Input: part model. Units: mm. Frame: model coordinates. Face numbers are marked on the shaded views. A direction names the side the tool comes from. Coordinates: 2 decimals unless noted, no trailing zeros. Write each loop counter-clockwise with the first axis right and the second up, starting at its lowest first coordinate (ties: lowest second). Pieces come first, ordered by that corner, then holes.
1) Section query B-B (y = -48). Output: boundary loops of the cut face in (x, z).
2) Section query D-D (z = -57.5). Output: boundary loops of the cut face in (x, y), then the cut area to 3 significant figures.
3) Set-up query: the marked faces 4, 5, 6 and 7. Return all of +Z, -Z, +X, -X, +Y, -Y with unobstructed straight access to the full face (end or side cutting, diameter ignored); none if empty.
4) Pin query (flat end, axial travel): pin 1 Ø1.5 at (y, z) = (-69, 32) entering from -X; pin 2 Ø3.5 at (x, y) = (-122, -49.5) entering from -Z; pin 3 Ø10 at (x, y) = (22.5, -47) entering from -Z. Return the tip coordinate at first contact, or that it passes through.
5) Draft query along X for the marked faces 1, 2 and 3. Return one class per face: pulls with the +X half, pulls with the -X half, needs draft (parallel to the pull), parting line crosses it, or undercut.
6) Section query A-A (z = 0). State how many separate pieces and enclosed holes the cut face has, then the cut area to 3 significant figures.
7) Line query: L1, parallel to Z at x = 14, y = -43.5; L2, parallel to Y at x = -47.5, z = 53; L3, parallel to X at y = -43.5, z = -13.5. Output: solid intervals per line, ascending.
8) Section query C-C (x = 51.5). Output: boundary loops of the cut face in (y, z), then the cut area to 3 significant figures.
from build123d import *

# Parameters (mm, degrees)
SKETCH_6_W                     = 111
SKETCH_6_H                     = 9
SKETCH_7_W                     = 12
SKETCH_7_H                     = 30
EXTRUDE_5_DEPTH                = 30
SKETCH_8_R                     = 3
CUT_EXTRUDE_2_DEPTH            = 200.07204757
FILLET_2_R                     = 6
SKETCH_9_W                     = 25.2
SKETCH_9_H                     = 33
CUT_EXTRUDE_3_DEPTH            = 178.121180423
PATTERN_START                  = -15
PATTERN_CIRCULAR_3_OUTLINE_R   = 3
PATTERN_CIRCULAR_3_DEPTH       = 30
PATTERN_START_2                = -37.701760736
PATTERN_CIRCULAR_3_2_OUTLINE_R = 3
PATTERN_CIRCULAR_3_2_DEPTH     = 30
PATTERN_CIRCULAR_3_3_OUTLINE_R = 3
PATTERN_CIRCULAR_3_3_DEPTH     = 0.833530395
PATTERN_CIRCULAR_3_4_OUTLINE_R = 3
PATTERN_CIRCULAR_3_4_DEPTH     = 30
PATTERN_CIRCULAR_3_5_OUTLINE_R = 3
PATTERN_CIRCULAR_3_5_DEPTH     = 0.833530395
PATTERN_START_3                = -16.5
PATTERN_CIRCULAR_3_6_OUTLINE_W = 25.2
PATTERN_CIRCULAR_3_6_OUTLINE_H = 9
PATTERN_CIRCULAR_3_6_DEPTH     = 33
PATTERN_START_4                = -38.368230341
PATTERN_CIRCULAR_3_7_OUTLINE_W = 25.2
PATTERN_CIRCULAR_3_7_OUTLINE_H = 9
PATTERN_CIRCULAR_3_7_DEPTH     = 33
PATTERN_CIRCULAR_3_8_OUTLINE_W = 25.2
PATTERN_CIRCULAR_3_8_OUTLINE_H = 9
PATTERN_CIRCULAR_3_8_DEPTH     = 33


# Read off the part's stored shape, not the designer's step: 阵列(圆周)3
with BuildPart() as part:
    # 草图6 → 旋转3 (revolve)
    with BuildSketch(Plane.XY, mode=Mode.PRIVATE) as revolve_3_sk:
        with Locations((31.774677383, -70.351637053)):
            Rectangle(SKETCH_6_W, SKETCH_6_H)
    revolve(revolve_3_sk.sketch.rotate(Axis((-23.725322617, -65.851637053, 0), (0, -1, 0)), 90), axis=Axis((-23.725322617, -65.851637053, 0), (0, -1, 0)))

    # 草图7 → 凸台-拉伸5 (add)
    with BuildSketch(Plane(origin=(0, -65.851637053, 0), x_dir=(1, 0, 0), z_dir=(0, 1, 0))):
        with Locations((69.274677383, 0)):
            Rectangle(SKETCH_7_W, SKETCH_7_H)
    extrude(amount=EXTRUDE_5_DEPTH)

    # 草图8 → 切除-拉伸2 (cut, through all)
    with BuildSketch(Plane.XY.offset(15)):
        with Locations((69.274677383, -41.851637053)):
            Circle(SKETCH_8_R)
        with Locations((69.274677383, -56.851637053)):
            Circle(SKETCH_8_R)
    extrude(amount=-CUT_EXTRUDE_2_DEPTH, mode=Mode.SUBTRACT)

    # 圆角2
    fillet_2_edges = [part.edges().sort_by_distance(p)[0] for p in [
        (63.274677383, -35.851637053, 0),
        (75.274677383, -35.851637053, 0),
    ]]
    fillet(fillet_2_edges, radius=FILLET_2_R - 0.0001)  # a hair under: the kernel refuses the full size

    # 草图9 → 切除-拉伸3 (cut, through all)
    with BuildSketch(Plane(origin=(0, -65.851637053, 0), x_dir=(1, 0, 0), z_dir=(0, 1, 0))):
        with Locations((48.274677383, 0)):
            Rectangle(SKETCH_9_W, SKETCH_9_H)
    extrude(amount=-CUT_EXTRUDE_3_DEPTH, mode=Mode.SUBTRACT)

    # 阵列(圆周)3 outline → 阵列(圆周)3 (add)
    with BuildSketch(Plane.XY.offset(PATTERN_START)):
        with BuildLine():
            ThreePointArc((-121.702148071, -35.851637053), (-125.944788758, -37.608996366), (-127.702148071, -41.851637053))
            Line((-127.702148071, -41.851637053), (-127.702148071, -65.851637053))
            Line((-127.702148071, -65.851637053), (-115.702148071, -65.851637053))
            Line((-115.702148071, -65.851637053), (-115.702148071, -41.851637053))
            ThreePointArc((-115.702148071, -41.851637053), (-117.459507384, -37.608996366), (-121.702148071, -35.851637053))
        make_face()
        with Locations((-119.777192079, -56.851637053)):
            Circle(PATTERN_CIRCULAR_3_OUTLINE_R, mode=Mode.SUBTRACT)
        with Locations((-119.777192079, -41.851637053)):
            Circle(PATTERN_CIRCULAR_3_OUTLINE_R, mode=Mode.SUBTRACT)
    extrude(amount=PATTERN_CIRCULAR_3_DEPTH)

    # Pattern Circular 3 2 outline → Pattern Circular 3 2 (add)
    # profile 1 of 2: a face of its own
    with BuildSketch(Plane(origin=(0, 0, 0), x_dir=(0.49999999999999767, 0, -0.86602540378444), z_dir=(0.8660254037844399, 0, 0.49999999999999795)).offset(PATTERN_START_2)):
        with BuildLine():
            Line((76.381545055, -65.851637053), (88.381545055, -65.851637053))
            Line((88.381545055, -65.851637053), (88.381545055, -41.851637053))
            ThreePointArc((88.381545055, -41.851637053), (86.624185742, -37.608996366), (82.381545055, -35.851637053))
            ThreePointArc((82.381545055, -35.851637053), (78.138904368, -37.608996366), (76.381545055, -41.851637053))
            Line((76.381545055, -41.851637053), (76.381545055, -65.851637053))
        make_face()
        with Locations((81.900306057, -56.851637053)):
            Circle(PATTERN_CIRCULAR_3_2_OUTLINE_R, mode=Mode.SUBTRACT)
        with Locations((81.900306057, -41.851637053)):
            Circle(PATTERN_CIRCULAR_3_2_OUTLINE_R, mode=Mode.SUBTRACT)
    # profile 2 of 2: a face of its own
    with BuildSketch(Plane(origin=(0, 0, 0), x_dir=(0.49999999999999767, 0, -0.86602540378444), z_dir=(0.8660254037844399, 0, 0.49999999999999795)).offset(PATTERN_START_2)):
        with BuildLine():
            Line((-114.595280399, -65.851637053), (-102.595280399, -65.851637053))
            Line((-102.595280399, -65.851637053), (-102.595280399, -41.851637053))
            ThreePointArc((-102.595280399, -41.851637053), (-104.352639712, -37.608996366), (-108.595280399, -35.851637053))
            ThreePointArc((-108.595280399, -35.851637053), (-112.837921086, -37.608996366), (-114.595280399, -41.851637053))
            Line((-114.595280399, -41.851637053), (-114.595280399, -65.851637053))
        make_face()
        with Locations((-107.151563405, -56.851637053)):
            Circle(PATTERN_CIRCULAR_3_2_OUTLINE_R, mode=Mode.SUBTRACT)
        with Locations((-107.151563405, -41.851637053)):
            Circle(PATTERN_CIRCULAR_3_2_OUTLINE_R, mode=Mode.SUBTRACT)
    extrude(amount=PATTERN_CIRCULAR_3_2_DEPTH)

    # Pattern Circular 3 3 outline → Pattern Circular 3 3 (add)
    with BuildSketch(Plane(origin=(0, 0, 0), x_dir=(0.49999999999999767, 0, -0.86602540378444), z_dir=(0.8660254037844399, 0, 0.49999999999999795)).offset(PATTERN_START_2)):
        with Locations((-107.151563405, -56.851637053)):
            Circle(PATTERN_CIRCULAR_3_3_OUTLINE_R)
        with Locations((-107.151563405, -41.851637053)):
            Circle(PATTERN_CIRCULAR_3_3_OUTLINE_R)
    extrude(amount=PATTERN_CIRCULAR_3_3_DEPTH)

    # Pattern Circular 3 4 outline → Pattern Circular 3 4 (add)
    # profile 1 of 2: a face of its own
    with BuildSketch(Plane(origin=(0, 0, 0), x_dir=(0.500000000000004, 0, 0.8660254037844363), z_dir=(0.8660254037844363, 0, -0.5000000000000042)).offset(PATTERN_START_2)):
        with BuildLine():
            Line((-102.595280399, 65.851637053), (-114.595280399, 65.851637053))
            Line((-114.595280399, 65.851637053), (-114.595280399, 41.851637053))
            ThreePointArc((-114.595280399, 41.851637053), (-112.837921086, 37.608996366), (-108.595280399, 35.851637053))
            ThreePointArc((-108.595280399, 35.851637053), (-104.352639712, 37.608996366), (-102.595280399, 41.851637053))
            Line((-102.595280399, 41.851637053), (-102.595280399, 65.851637053))
        make_face()
        with Locations((-107.151563405, 41.851637053)):
            Circle(PATTERN_CIRCULAR_3_4_OUTLINE_R, mode=Mode.SUBTRACT)
        with Locations((-107.151563405, 56.851637053)):
            Circle(PATTERN_CIRCULAR_3_4_OUTLINE_R, mode=Mode.SUBTRACT)
    # profile 2 of 2: a face of its own
    with BuildSketch(Plane(origin=(0, 0, 0), x_dir=(0.500000000000004, 0, 0.8660254037844363), z_dir=(0.8660254037844363, 0, -0.5000000000000042)).offset(PATTERN_START_2)):
        with BuildLine():
            Line((88.381545055, 65.851637053), (76.381545055, 65.851637053))
            Line((76.381545055, 65.851637053), (76.381545055, 41.851637053))
            ThreePointArc((76.381545055, 41.851637053), (78.138904368, 37.608996366), (82.381545055, 35.851637053))
            ThreePointArc((82.381545055, 35.851637053), (86.624185742, 37.608996366), (88.381545055, 41.851637053))
            Line((88.381545055, 41.851637053), (88.381545055, 65.851637053))
        make_face()
        with Locations((81.900306057, 41.851637053)):
            Circle(PATTERN_CIRCULAR_3_4_OUTLINE_R, mode=Mode.SUBTRACT)
        with Locations((81.900306057, 56.851637053)):
            Circle(PATTERN_CIRCULAR_3_4_OUTLINE_R, mode=Mode.SUBTRACT)
    extrude(amount=PATTERN_CIRCULAR_3_4_DEPTH)

    # Pattern Circular 3 5 outline → Pattern Circular 3 5 (add)
    with BuildSketch(Plane(origin=(0, 0, 0), x_dir=(0.500000000000004, 0, 0.8660254037844363), z_dir=(0.8660254037844363, 0, -0.5000000000000042)).offset(PATTERN_START_2)):
        with Locations((81.900306057, 56.851637053)):
            Circle(PATTERN_CIRCULAR_3_5_OUTLINE_R)
        with Locations((81.900306057, 41.851637053)):
            Circle(PATTERN_CIRCULAR_3_5_OUTLINE_R)
    extrude(amount=PATTERN_CIRCULAR_3_5_DEPTH)

    # Pattern Circular 3 6 outline → Pattern Circular 3 6 (cut)
    with BuildSketch(Plane.XY.offset(PATTERN_START_3)):
        with Locations((-98.777192079, -70.351637053)):
            Rectangle(PATTERN_CIRCULAR_3_6_OUTLINE_W, PATTERN_CIRCULAR_3_6_OUTLINE_H)
    extrude(amount=PATTERN_CIRCULAR_3_6_DEPTH, mode=Mode.SUBTRACT)

    # Pattern Circular 3 7 outline → Pattern Circular 3 7 (cut)
    with BuildSketch(Plane(origin=(0, 0, 0), x_dir=(0.49999999999999767, 0, -0.86602540378444), z_dir=(0.8660254037844399, 0, 0.49999999999999795)).offset(PATTERN_START_4)):
        with Locations((60.900306057, -70.351637053)):
            Rectangle(PATTERN_CIRCULAR_3_7_OUTLINE_W, PATTERN_CIRCULAR_3_7_OUTLINE_H)
        with Locations((-86.151563405, -70.351637053)):
            Rectangle(PATTERN_CIRCULAR_3_7_OUTLINE_W, PATTERN_CIRCULAR_3_7_OUTLINE_H)
    extrude(amount=PATTERN_CIRCULAR_3_7_DEPTH, mode=Mode.SUBTRACT)

    # Pattern Circular 3 8 outline → Pattern Circular 3 8 (cut)
    with BuildSketch(Plane(origin=(0, 0, 0), x_dir=(0.500000000000004, 0, 0.8660254037844363), z_dir=(0.8660254037844363, 0, -0.5000000000000042)).offset(PATTERN_START_4)):
        with Locations((-86.151563405, 70.351637053)):
            Rectangle(PATTERN_CIRCULAR_3_8_OUTLINE_W, PATTERN_CIRCULAR_3_8_OUTLINE_H)
        with Locations((60.900306057, 70.351637053)):
            Rectangle(PATTERN_CIRCULAR_3_8_OUTLINE_W, PATTERN_CIRCULAR_3_8_OUTLINE_H)
    extrude(amount=PATTERN_CIRCULAR_3_8_DEPTH, mode=Mode.SUBTRACT)


solid = part.part
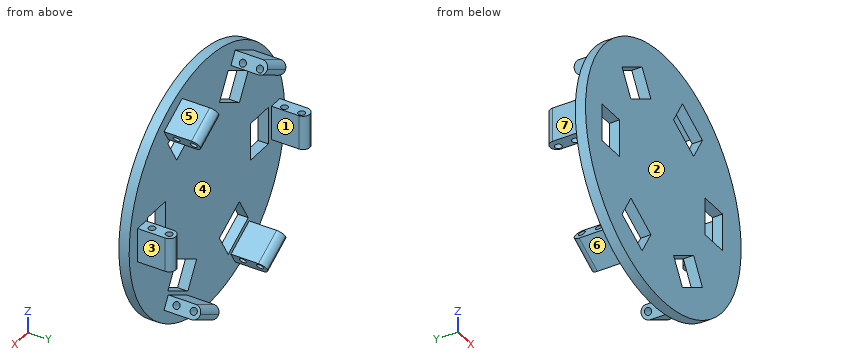
Answer:
1. outline: (-127.7, -15) - (-115.7, -15) - (-115.7, 15) - (-127.7, 15) - close; (-89.95, -80.39) - (-63.97, -95.39) - (-57.97, -85) - (-83.95, -70) - close; (-89.95, 80.39) - (-83.95, 70) - (-57.97, 85) - (-63.97, 95.39) - close; (5.54, -85) - (11.54, -95.39) - (37.52, -80.39) - (31.52, -70) - close; (5.54, 85) - (31.52, 70) - (37.52, 80.39) - (11.54, 95.39) - close; (63.27, -15) - (75.27, -15) - (75.27, 15) - (63.27, 15) - close
2. outline: (-118.67, -74.85) - (-77.5, -74.85) - (-77.5, -65.85) - (-118.67, -65.85) - close; (-47.51, -74.85) - (-2.99, -74.85) - (-2.99, -65.85) - (-47.51, -65.85) - close; (27, -74.85) - (71.22, -74.85) - (71.22, -65.85) - (27, -65.85) - close
2. area: 1,170 mm2
3. face 4: +Y
3. face 5: +Z, +X, +Y
3. face 6: -Z, -X, +Y
3. face 7: +Z, -Z, -X, +Y
4. pin 1: stops at x = -130.24
4. pin 2: stops at z = -15
4. pin 3: stops at z = -91.95
5. face 1: undercut
5. face 2: needs draft
5. face 3: pulls with the +X half
6. separate pieces: 3
6. enclosed holes: 4
6. area: 2,120 mm2
7. L1: z = -93.97 to -89.38, -83.59 to -80.11, 80.11 to 83.59, 89.38 to 93.97
7. L2: y = -74.85 to -65.85
7. L3: x = -127.7 to -122.28, -117.27 to -115.7, 63.27 to 66.77, 71.78 to 75.27
8. outline: (-74.85, -81.62) - (-65.85, -81.62) - (-65.85, -16.5) - (-74.85, -16.5) - close; (-74.85, 16.5) - (-65.85, 16.5) - (-65.85, 81.62) - (-74.85, 81.62) - close
8. area: 1,170 mm2
